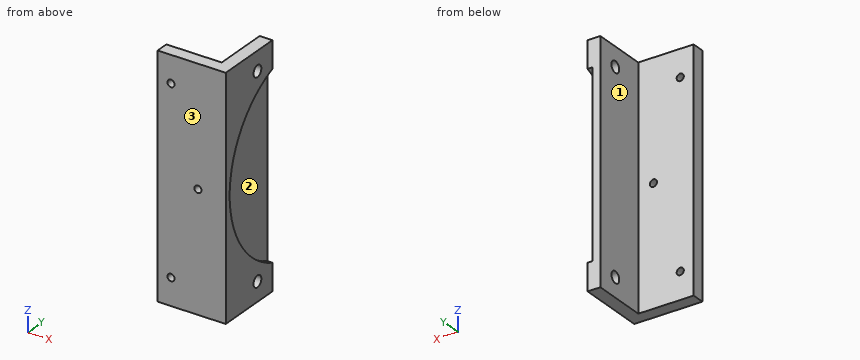
```python
from build123d import *

# Parameters (mm, degrees)
BOSS_EXTRUDE1_DEPTH          = 190
SKETCH3_R                    = 72.75
CUT_EXTRUDE3_DEPTH           = 3.5
CUT_EXTRUDE4_DEPTH           = 7.05
CUT_EXTRUDE5_DEPTH           = 7.05
TAP_DRILL_FOR_M10X1_5_TAP1_D = 8.5
CUT_EXTRUDE6_REACH           = 191.26
SKETCH8_R                    = 2.665


with BuildPart() as part:
    # Sketch1 → Boss-Extrude1 (new body)
    with BuildSketch(Plane.XY):
        Polygon((-25.4, -25.4), (25.4, -25.4), (25.4, 25.4), (15.875, 25.4), (15.875, -15.875), (-25.4, -15.875), align=None)
    extrude(amount=BOSS_EXTRUDE1_DEPTH)

    # Sketch3 → Cut-Extrude3 (cut)
    with BuildSketch(Plane(origin=(25.4, 0, 0), x_dir=(0, 0, -1), z_dir=(1, 0, 0))):
        with Locations((-95, 51.6)):
            Circle(SKETCH3_R)
    extrude(amount=-CUT_EXTRUDE3_DEPTH, mode=Mode.SUBTRACT)

    # Sketch4 → Cut-Extrude4 (cut)
    with BuildSketch(Plane.XY.offset(190)):
        Polygon((25.4, -25.4), (25.4, 25.4), (15.875, 25.4), (15.875, -15.875), (-25.4, -15.875), (-25.4, -25.4), align=None)
    extrude(amount=-CUT_EXTRUDE4_DEPTH, mode=Mode.SUBTRACT)

    # Sketch5 → Cut-Extrude5 (cut)
    with BuildSketch(Plane(origin=(0, 0, 0), x_dir=(-1, 0, 0), z_dir=(0, 0, -1))):
        Polygon((-25.4, 25.4), (-25.4, -25.4), (25.4, -25.4), (25.4, -15.875), (-15.875, -15.875), (-15.875, 25.4), align=None)
    extrude(amount=-CUT_EXTRUDE5_DEPTH, mode=Mode.SUBTRACT)

    # Tap Drill for M10x1.5 Tap1 (through all)
    with Locations(Plane(origin=(25.4, 9.1, 168.612159322), x_dir=(0, 0, 1), z_dir=(1, 0, 0))):
        with Locations((0, 0), (-147.224318644, 0)):
            Hole(TAP_DRILL_FOR_M10X1_5_TAP1_D / 2)

    # Sketch8 → Cut-Extrude6 (cut, up to next)
    with BuildSketch(Plane(origin=(0, -15.875, 0), x_dir=(1, 0, 0), z_dir=(0, 1, 0)), mode=Mode.PRIVATE) as cut_extrude6_sk1:
        with Locations(Location((-15.4, -27.05, 0), (0, 0, 270))):
            Circle(SKETCH8_R)
    cut_extrude6_tool1 = extrude(cut_extrude6_sk1.sketch, amount=-CUT_EXTRUDE6_REACH, mode=Mode.PRIVATE) & part.part
    # Sketch8 → Cut-Extrude6 (cut, up to next)
    with BuildSketch(Plane(origin=(0, -15.875, 0), x_dir=(1, 0, 0), z_dir=(0, 1, 0)), mode=Mode.PRIVATE) as cut_extrude6_sk2:
        with Locations(Location((4.6, -95, 0), (0, 0, 270))):
            Circle(SKETCH8_R)
    cut_extrude6_tool2 = extrude(cut_extrude6_sk2.sketch, amount=-CUT_EXTRUDE6_REACH, mode=Mode.PRIVATE) & part.part
    # Sketch8 → Cut-Extrude6 (cut, up to next)
    with BuildSketch(Plane(origin=(0, -15.875, 0), x_dir=(1, 0, 0), z_dir=(0, 1, 0)), mode=Mode.PRIVATE) as cut_extrude6_sk3:
        with Locations(Location((-15.4, -162.95, 0), (0, 0, 270))):
            Circle(SKETCH8_R)
    cut_extrude6_tool3 = extrude(cut_extrude6_sk3.sketch, amount=-CUT_EXTRUDE6_REACH, mode=Mode.PRIVATE) & part.part
    add(cut_extrude6_tool1.solids().sort_by_distance((-15.4, -15.875, 27.05))[0], mode=Mode.SUBTRACT)
    add(cut_extrude6_tool2.solids().sort_by_distance((4.6, -15.875, 95))[0], mode=Mode.SUBTRACT)
    add(cut_extrude6_tool3.solids().sort_by_distance((-15.4, -15.875, 162.95))[0], mode=Mode.SUBTRACT)


solid = part.part
```
Work out the finished part from the listing and answer in its coordinate system (mm). Face numbers are marked on the shaded views. A direction names the side the tool comes from. Round coordinates to 2 decimals unless told otherwise and drop trailing zeros. Order: outer loops, then holes, each group sorted by start corner. A loop starts at its lowest first (then second) coordinate and runs counter-clockwise, first axis right, second up.
Q1. A tool of negligible diameter and unlimited length cuts with its end or side. For the marked faces 1, 2 and 3, from which of +Z, -Z, +X, -X, +Y, -Y can it reach the whole face along a straight path? Write none if from no direction.
Solution:
face 1: +Z, -Z, -X, +Y
face 2: +X, +Y
face 3: +Z, -Z, +X, -X, -Y
Q2. A cutting plane is placed at D-D, the plane y = 9.1. Determine the outline of the cut face in (x, z) (3 decimals).
Solution:
outline: (15.875, 7.05) - (25.4, 7.05) - (25.4, 17.138) - (15.875, 17.138) - close; (15.875, 25.638) - (25.4, 25.638) - (25.4, 35.955) - (21.9, 35.955) - (21.9, 154.045) - (25.4, 154.045) - (25.4, 164.362) - (15.875, 164.362) - close; (15.875, 172.862) - (25.4, 172.862) - (25.4, 182.95) - (15.875, 182.95) - close
Q3. A cutting plane is placed at A-A, the plane x = 4.6. Determine the outline of the cut face in (y, z) (3 decimals), then the cut area to 3 significant figures.
Solution:
outline: (-25.4, 7.05) - (-15.875, 7.05) - (-15.875, 92.335) - (-25.4, 92.335) - close; (-25.4, 97.665) - (-15.875, 97.665) - (-15.875, 182.95) - (-25.4, 182.95) - close
area: 1,620 mm2
Q4. Given pin 1 Ø12.5 at (x, z) = (-12, 86.5) entering from +Y (3 decimals); pin 2 Ø8 at (y, z) = (-12, 88) entering from +X; pin 3 Ø10 at (y, z) = (9.1, 21.39) entering from -X (3 decimals), each flat-ended and moving along its own axis, determine where each tip first touches the part or whether it passes through.
Solution:
pin 1: stops at y = -15.875
pin 2: stops at x = 21.9
pin 3: stops at x = 15.875
Q5. A cutting plane is placed at B-B, the plane x = -15.4. Determine the outline of the cut face in (y, z) (3 decimals), then the cut area to 3 significant figures.
Solution:
outline: (-25.4, 7.05) - (-15.875, 7.05) - (-15.875, 24.385) - (-25.4, 24.385) - close; (-25.4, 29.715) - (-15.875, 29.715) - (-15.875, 160.285) - (-25.4, 160.285) - close; (-25.4, 165.615) - (-15.875, 165.615) - (-15.875, 182.95) - (-25.4, 182.95) - close
area: 1,570 mm2
Q6. A cutting plane is placed at C-C, the plane z = 95. Determine the outline of the cut face in (x, y) (3 decimals), then the cut area to 3 significant figures.
Solution:
outline: (-25.4, -25.4) - (1.935, -25.4) - (1.935, -15.875) - (-25.4, -15.875) - close; (7.265, -25.4) - (25.4, -25.4) - (25.4, -21.15) - (21.9, -21.15) - (21.9, 25.4) - (15.875, 25.4) - (15.875, -15.875) - (7.265, -15.875) - close
area: 663 mm2
Q7. Find the intervals of material crossed by line 1 along Z through (x, y) = (23, 9); line 2 along Y through (x, z) = (15.5, 147) (3 decimals); line 3 along X through (y, z) = (-23.25, 95) (3 decimals), in increasing order.
Solution:
line 1: z = 7.05 to 17.14, 25.64 to 36.03, 153.97 to 164.36, 172.86 to 182.95
line 2: y = -25.4 to -15.875
line 3: x = -25.4 to 1.935, 7.265 to 25.4
